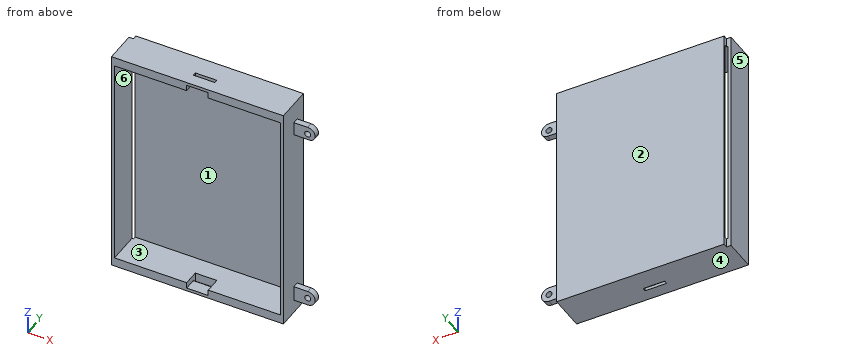
```python
from build123d import *

# Parameters (mm, degrees)
SKETCH1_R                = 1
SKETCH1_W                = 55.4
SKETCH1_H                = 71.4
BOSS_EXTRUDE1_DEPTH      = 5
SKETCH2_W                = 55.4
SKETCH2_H                = 71.4
BOSS_EXTRUDE2_DEPTH      = 1.5
SKETCH4_W                = 7.703515063
SKETCH4_H                = 8.608986158
CUT_EXTRUDE1_DEPTH       = 105.5
MOVE_FACE1_BY            = 7
MOVE_FACE2_BY            = 7.5
MOVE_FACE3_BY            = 4
MOVE_FACE3_2_BY          = 4
MOVE_FACE4_BY            = 4
MOVE_FACE4_2_BY          = 4
MOVE_FACE5_BY            = 0.4
MOVE_FACE5_2_BY          = 0.4
MOVE_FACE6_BY            = 0.4
MOVE_FACE6_2_BY          = 0.4
MOVE_START               = 3
MOVE_FACE7_OUTLINE_W     = 58.4
MOVE_FACE7_OUTLINE_H     = 74.4
MOVE_FACE7_OUTLINE_W_2   = 55.4
MOVE_FACE7_OUTLINE_H_2   = 71.4
MOVE_FACE7_DEPTH         = 2
MOVE_START_2             = -25.141552832
MOVE_FACE8_OUTLINE_W     = 0.5
MOVE_FACE8_OUTLINE_H     = 10
MOVE_FACE8_DEPTH         = 56
MOVE_START_3             = -33.2
MOVE_FACE8_2_OUTLINE_W   = 58.4
MOVE_FACE8_2_OUTLINE_H   = 10
MOVE_FACE8_2_DEPTH       = 0.5
MOVE_START_4             = 40.7
MOVE_FACE8_3_OUTLINE_W   = 58.4
MOVE_FACE8_3_OUTLINE_H   = 10
MOVE_FACE8_3_DEPTH       = 0.5
MOVE_START_5             = -32.7
MOVE_FACE8_4_OUTLINE_W   = 0.5
MOVE_FACE8_4_OUTLINE_H   = 10
MOVE_FACE8_4_OUTLINE_H_2 = 1
MOVE_FACE8_4_DEPTH       = 73.4
MOVE_START_6             = 35.858447168
MOVE_FACE8_5_OUTLINE_W   = 0.5
MOVE_FACE8_5_OUTLINE_H   = 9
MOVE_FACE8_5_DEPTH       = 4.841552832
MOVE_FACE8_6_OUTLINE_W   = 0.5
MOVE_FACE8_6_OUTLINE_H   = 9
MOVE_FACE8_6_DEPTH       = 2.558447168
CUT_EXTRUDE2_DEPTH       = 66
CUT_EXTRUDE2_DEPTH_BACK  = 64
SKETCH5_W                = 9.341764375
SKETCH5_H                = 8.237393027
CUT_EXTRUDE3_DEPTH       = 4
FILLET3_R                = 2
MOVE_FACE9_OUTLINE_W     = 57.4
MOVE_FACE9_OUTLINE_H     = 73.4
MOVE_FACE9_OUTLINE_W_2   = 55.4
MOVE_FACE9_OUTLINE_H_2   = 71.4
MOVE_FACE9_DEPTH         = 2.5
SKETCH7_W                = 57.4
SKETCH7_H                = 73.4
BOSS_EXTRUDE3_DEPTH      = 0.5
SKETCH8_W                = 57.4
SKETCH8_H                = 73.4
CUT_EXTRUDE4_DEPTH       = 1
MOVE_FACE10_BY           = 0.25
MOVE_FACE10_2_BY         = 0.25
MOVE_FACE11_BY           = 0.25
MOVE_FACE11_2_BY         = 0.25
SKETCH9_W                = 1.5
SKETCH9_H                = 73.4
CUT_EXTRUDE5_DEPTH       = 1.5
MOVE_START_7             = -34.7
MOVE_FACE12_DEPTH        = 2
MOVE_FACE12_2_DEPTH      = 2
CUT_EXTRUDE6_DEPTH       = 5.2
SKETCH12_W               = 7.2
SKETCH12_H               = 1.2
CUT_EXTRUDE7_DEPTH       = 108.2


# Read off the part's stored shape, not the designer's step: Move Face7, Move Face8, Move Face9, Move Face12
with BuildPart() as part:
    # Sketch1 → Boss-Extrude1 (new body)
    with BuildSketch(Plane(origin=(0, 0, 0), x_dir=(1, 0, 0), z_dir=(0, 1, 0))):
        with BuildLine():
            Line((26.077909727, -37.2), (26.077909727, -35.858447168))
            Line((26.077909727, -35.858447168), (29.822090273, -35.858447168))
            ThreePointArc((29.822090273, -35.858447168), (32.322090273, -33.358447168), (29.822090273, -30.858447168))
            Line((29.822090273, -30.858447168), (26.077909727, -30.858447168))
            Line((26.077909727, -30.858447168), (26.077909727, 25.141552832))
            Line((26.077909727, 25.141552832), (29.822090273, 25.141552832))
            ThreePointArc((29.822090273, 25.141552832), (32.322090273, 27.641552832), (29.822090273, 30.141552832))
            Line((29.822090273, 30.141552832), (26.077909727, 30.141552832))
            Line((26.077909727, 30.141552832), (26.077909727, 37.2))
            Line((26.077909727, 37.2), (-32.322090273, 37.2))
            Line((-32.322090273, 37.2), (-32.322090273, -37.2))
            Line((-32.322090273, -37.2), (26.077909727, -37.2))
        make_face()
        with Locations(Location((29.822090273, 27.641552832, 0), (0, 0, 270))):
            Circle(SKETCH1_R, mode=Mode.SUBTRACT)
        with Locations(Location((29.822090273, -33.358447168, 0), (0, 0, 270))):
            Circle(SKETCH1_R, mode=Mode.SUBTRACT)
        with Locations((-3.122090273, 0)):
            Rectangle(SKETCH1_W, SKETCH1_H, mode=Mode.SUBTRACT)
    extrude(amount=BOSS_EXTRUDE1_DEPTH)

    # Sketch2 → Boss-Extrude2 (add)
    with BuildSketch(Plane(origin=(0, 0, 0), x_dir=(1, 0, 0), z_dir=(0, 1, 0))):
        with Locations((-3.122090273, 0)):
            Rectangle(SKETCH2_W, SKETCH2_H)
    extrude(amount=BOSS_EXTRUDE2_DEPTH)

    # Sketch4 → Cut-Extrude1 (cut)
    with BuildSketch(Plane.XY.offset(35.858447168)):
        with Locations((29.929667259, 6.304493079)):
            Rectangle(SKETCH4_W, SKETCH4_H)
    extrude(amount=-CUT_EXTRUDE1_DEPTH, mode=Mode.SUBTRACT)

    # Move Face1: a face moved outward by 7.0
    extrude(part.faces().sort_by_distance((-2.752621979, 0, 0.033029774))[0], amount=MOVE_FACE1_BY, dir=(0, -1, 0))

    # Move Face2: a face moved inward by 7.5
    extrude(part.faces().sort_by_distance((-3.122090273, 1.5, 0))[0], amount=MOVE_FACE2_BY, dir=(0, -1, 0), mode=Mode.SUBTRACT)

    # Move Face3: a face moved outward by 4.0
    extrude(part.faces().sort_by_distance((-3.122090273, -1, 37.2))[0], amount=MOVE_FACE3_BY, dir=(0, 0, 1))

    # Move Face3 2: a face moved outward by 4.0
    extrude(part.faces().sort_by_distance((-3.122090273, -0.5, -35.7))[0], amount=MOVE_FACE3_2_BY, dir=(0, 0, 1))

    # Move Face4: a face moved inward by 4.0
    extrude(part.faces().sort_by_distance((-3.122090273, -0.5, 35.7))[0], amount=MOVE_FACE4_BY, dir=(0, 0, 1), mode=Mode.SUBTRACT)

    # Move Face4 2: a face moved inward by 4.0
    extrude(part.faces().sort_by_distance((-3.122090273, -1, -37.2))[0], amount=MOVE_FACE4_2_BY, dir=(0, 0, 1), mode=Mode.SUBTRACT)

    # Move Face5: a face moved outward by 0.4
    extrude(part.faces().sort_by_distance((24.577909727, -0.5, 4))[0], amount=MOVE_FACE5_BY, dir=(-1, 0, 0))

    # Move Face5 2: a face moved outward by 0.4
    extrude(part.faces().sort_by_distance((-32.322090273, -1, 4))[0], amount=MOVE_FACE5_2_BY, dir=(-1, 0, 0))

    # Move Face6: a face moved inward by 0.4
    extrude(part.faces().sort_by_distance((-30.822090273, -0.5, 4))[0], amount=MOVE_FACE6_BY, dir=(-1, 0, 0), mode=Mode.SUBTRACT)

    # Move Face6 2: a face moved inward by 0.4
    extrude(part.faces().sort_by_distance((26.077909727, -0.831838565, 4.127976775))[0], amount=MOVE_FACE6_2_BY, dir=(-1, 0, 0), mode=Mode.SUBTRACT)

    # Move Face7 outline → Move Face7 (cut)
    with BuildSketch(Plane(origin=(0, 0, 0), x_dir=(1, 0, 0), z_dir=(0, 1, 0)).offset(MOVE_START)):
        with Locations((-3.522090273, -4)):
            Rectangle(MOVE_FACE7_OUTLINE_W, MOVE_FACE7_OUTLINE_H)
        with Locations((-3.522090273, -4)):
            Rectangle(MOVE_FACE7_OUTLINE_W_2, MOVE_FACE7_OUTLINE_H_2, mode=Mode.SUBTRACT)
    extrude(amount=MOVE_FACE7_DEPTH, mode=Mode.SUBTRACT)

    # Move Face8 outline → Move Face8 (cut)
    with BuildSketch(Plane.XY.offset(MOVE_START_2)):
        with Locations((-32.472090273, -2)):
            Rectangle(MOVE_FACE8_OUTLINE_W, MOVE_FACE8_OUTLINE_H)
        with Locations((25.427909727, -2)):
            Rectangle(MOVE_FACE8_OUTLINE_W, MOVE_FACE8_OUTLINE_H)
    extrude(amount=MOVE_FACE8_DEPTH, mode=Mode.SUBTRACT)

    # Move Face8 2 outline → Move Face8 2 (cut)
    with BuildSketch(Plane.XY.offset(MOVE_START_3)):
        with Locations((-3.522090273, -2)):
            Rectangle(MOVE_FACE8_2_OUTLINE_W, MOVE_FACE8_2_OUTLINE_H)
    extrude(amount=MOVE_FACE8_2_DEPTH, mode=Mode.SUBTRACT)

    # Move Face8 3 outline → Move Face8 3 (cut)
    with BuildSketch(Plane.XY.offset(MOVE_START_4)):
        with Locations((-3.522090273, -2)):
            Rectangle(MOVE_FACE8_3_OUTLINE_W, MOVE_FACE8_3_OUTLINE_H)
    extrude(amount=MOVE_FACE8_3_DEPTH, mode=Mode.SUBTRACT)

    # Move Face8 4 outline → Move Face8 4 (cut)
    with BuildSketch(Plane.XY.offset(MOVE_START_5)):
        with Locations((-32.472090273, -2)):
            Rectangle(MOVE_FACE8_4_OUTLINE_W, MOVE_FACE8_4_OUTLINE_H)
        with Locations((25.427909727, 2.5)):
            Rectangle(MOVE_FACE8_4_OUTLINE_W, MOVE_FACE8_4_OUTLINE_H_2)
    extrude(amount=MOVE_FACE8_4_DEPTH, mode=Mode.SUBTRACT)

    # Move Face8 5 outline → Move Face8 5 (cut)
    with BuildSketch(Plane.XY.offset(MOVE_START_6)):
        with Locations((25.427909727, -2.5)):
            Rectangle(MOVE_FACE8_5_OUTLINE_W, MOVE_FACE8_5_OUTLINE_H)
    extrude(amount=MOVE_FACE8_5_DEPTH, mode=Mode.SUBTRACT)

    # Move Face8 6 outline → Move Face8 6 (cut)
    with BuildSketch(Plane.XY.offset(MOVE_START_5)):
        with Locations((25.427909727, -2.5)):
            Rectangle(MOVE_FACE8_6_OUTLINE_W, MOVE_FACE8_6_OUTLINE_H)
    extrude(amount=MOVE_FACE8_6_DEPTH, mode=Mode.SUBTRACT)

    # Sketch5 → Cut-Extrude2 (cut, two sides: drawn at the far end of the back side and taken through both)
    with BuildSketch(Plane.XY.offset(-CUT_EXTRUDE2_DEPTH_BACK)):
        with Locations((29.848791915, -4.118696514)):
            Rectangle(SKETCH5_W, SKETCH5_H)
    extrude(amount=CUT_EXTRUDE2_DEPTH + CUT_EXTRUDE2_DEPTH_BACK, mode=Mode.SUBTRACT)

    # Sketch6 → Cut-Extrude3 (cut)
    with BuildSketch(Plane(origin=(0, 2, 0), x_dir=(1, 0, 0), z_dir=(0, 1, 0))):
        Polygon((25.177909727, -30.858447168), (25.177909727, -31.358447168), (32.688438313, -31.358447168), (32.688438313, -30.19770306), (25.177909727, -30.19770306), align=None)
    extrude(amount=-CUT_EXTRUDE3_DEPTH, mode=Mode.SUBTRACT)

    # Fillet3
    fillet3_edges = [part.edges().sort_by_distance(p)[0] for p in [
        (31.322090273, 1, 31.358447168),
    ]]
    fillet(fillet3_edges, radius=FILLET3_R)

    # Move Face9 outline → Move Face9 (add)
    with BuildSketch(Plane(origin=(0, 0, 0), x_dir=(1, 0, 0), z_dir=(0, 1, 0)).offset(MOVE_START)):
        with Locations((-3.522090273, -4)):
            Rectangle(MOVE_FACE9_OUTLINE_W, MOVE_FACE9_OUTLINE_H)
        with Locations((-3.522090273, -4)):
            Rectangle(MOVE_FACE9_OUTLINE_W_2, MOVE_FACE9_OUTLINE_H_2, mode=Mode.SUBTRACT)
    extrude(amount=MOVE_FACE9_DEPTH)

    # Sketch7 → Boss-Extrude3 (add)
    with BuildSketch(Plane(origin=(0, 5.5, 0), x_dir=(1, 0, 0), z_dir=(0, 1, 0))):
        with Locations((-3.522090273, -4)):
            Rectangle(SKETCH7_W, SKETCH7_H)
    extrude(amount=BOSS_EXTRUDE3_DEPTH)

    # Sketch8 → Cut-Extrude4 (cut)
    with BuildSketch(Plane.XZ.offset(7)):
        with Locations((-3.522090273, 4)):
            Rectangle(SKETCH8_W, SKETCH8_H)
    extrude(amount=-CUT_EXTRUDE4_DEPTH, mode=Mode.SUBTRACT)

    # Move Face10: a face moved inward by 0.25
    extrude(part.faces().sort_by_distance((28.366938403, 0, -27.641552832))[0], amount=MOVE_FACE10_BY, dir=(0, 1, 0), mode=Mode.SUBTRACT)

    # Move Face10 2: a face moved inward by 0.25
    extrude(part.faces().sort_by_distance((28.373500925, 0, 33.610852536))[0], amount=MOVE_FACE10_2_BY, dir=(0, 1, 0), mode=Mode.SUBTRACT)

    # Move Face11: a face moved outward by 0.25
    extrude(part.faces().sort_by_distance((28.373500925, 2, 33.610852536))[0], amount=MOVE_FACE11_BY, dir=(0, 1, 0))

    # Move Face11 2: a face moved outward by 0.25
    extrude(part.faces().sort_by_distance((28.366938403, 2, -27.641552832))[0], amount=MOVE_FACE11_2_BY, dir=(0, 1, 0))

    # Sketch9 → Cut-Extrude5 (cut)
    with BuildSketch(Plane(origin=(0, 6, 0), x_dir=(1, 0, 0), z_dir=(0, 1, 0))):
        with Locations((-31.472090273, -4)):
            Rectangle(SKETCH9_W, SKETCH9_H)
    extrude(amount=-CUT_EXTRUDE5_DEPTH, mode=Mode.SUBTRACT)

    # Move Face12 outline → Move Face12 (add)
    with BuildSketch(Plane.XY.offset(MOVE_START_7)):
        Polygon((-32.222090273, 4.5), (-32.222090273, -6), (25.177909727, -6), (25.177909727, 6), (-30.722090273, 6), (-30.722090273, 4.5), align=None)
    extrude(amount=MOVE_FACE12_DEPTH)

    # Move Face12 2 outline → Move Face12 2 (add)
    with BuildSketch(Plane.XY.offset(MOVE_START_4)):
        Polygon((-32.222090273, 4.5), (-32.222090273, -6), (25.177909727, -6), (25.177909727, 6), (-30.722090273, 6), (-30.722090273, 4.5), align=None)
    extrude(amount=MOVE_FACE12_2_DEPTH)

    # Sketch10 → Cut-Extrude6 (cut)
    with BuildSketch(Plane.XZ.offset(6)):
        Polygon((-3.522090273, 41.7), (0.077909727, 41.7), (0.077909727, 38.920271818), (-7.122090273, 38.920271818), (-7.122090273, 41.7), align=None)
        Polygon((-7.122090273, -33.7), (-3.522090273, -33.7), (0.077909727, -33.7), (0.077909727, -30.920271818), (-7.122090273, -30.920271818), align=None)
    extrude(amount=-CUT_EXTRUDE6_DEPTH, mode=Mode.SUBTRACT)

    # Sketch12 → Cut-Extrude7 (cut)
    with BuildSketch(Plane.XY.offset(42.7)):
        with Locations((-3.522090273, -1.4)):
            Rectangle(SKETCH12_W, SKETCH12_H)
    extrude(amount=-CUT_EXTRUDE7_DEPTH, mode=Mode.SUBTRACT)


solid = part.part
```
Source: CAD feature listing. Evaluate the final solid. Frame: model axes, mm. Face numbers are marked on the shaded views. A direction names the side the tool comes from. Give positions to 0.01 mm unless a question says otherwise; leave off trailing zeros. Order: outer loops, then holes, each group sorted by start corner. A loop starts at its lowest first (then second) coordinate and runs counter-clockwise, first axis right, second up. Notation, with made-up numbers: (26, -31) -> (61, -31) arc R29 cw to (61, -9) -> close; hole circle Ø6 at (72.5, 36.25). An arc over 180 degrees is marked (long way). Use a Markdown table: item, result.
Q1. Section D-D (x = -6). Return the cut outline in (y, z), and give its area (3 significant figures).
A:
| item | result |
|---|---|
| outline | (-6, -34.7) -> (-2, -34.7) -> (-2, -33.7) -> (-6, -33.7) -> close; (-6, 41.7) -> (-2, 41.7) -> (-2, 42.7) -> (-6, 42.7) -> close; (-0.8, -34.7) -> (6, -34.7) -> (6, 42.7) -> (-0.8, 42.7) -> (-0.8, 39.7) -> (5.5, 39.7) -> (5.5, -31.7) -> (-0.8, -31.7) -> close |
| area | 84.5 mm^2 |
Q2. Access query for the marked faces 5 and 6. Directions: +Z, -Z, +X, -X, +Y, -Y. A direction counts if a zero-diameter tool reaches every point of the face in a straight line with its end or side. Return the directions, or none.
A:
| item | result |
|---|---|
| face 5 | +Z, -Z, -X, +Y, -Y |
| face 6 | +Y, -Y |
Q3. Section B-B (y = -3.75). Return the cut outline in (x, z), and give its area (3 significant figures).
A:
| item | result |
|---|---|
| outline | (-32.22, -34.7) -> (25.18, -34.7) -> (25.18, 42.7) -> (-32.22, 42.7) -> close; hole (-31.22, -31.7) -> (-7.12, -31.7) -> (-7.12, -33.7) -> (0.08, -33.7) -> (0.08, -31.7) -> (24.18, -31.7) -> (24.18, 39.7) -> (0.08, 39.7) -> (0.08, 41.7) -> (-7.12, 41.7) -> (-7.12, 39.7) -> (-31.22, 39.7) -> close |
| area | 458 mm^2 |
Q4. Section A-A (x = 26). Return the cut outline in (y, z).
A:
| item | result |
|---|---|
| outline | (0.25, -30.14) -> (2.25, -30.14) -> (2.25, -25.14) -> (0.25, -25.14) -> close; (0.25, 31.36) -> (2.25, 31.36) -> (2.25, 35.86) -> (0.25, 35.86) -> close |
Q5. Pull-direction query (Z, two-part tool) for the marked faces 1, 2, 3 and 4; classes: +Z half, -Z half, draft (parallel to the pull), parting line (faces both ways), or undercut.
A:
| item | result |
|---|---|
| face 1 | undercut |
| face 2 | draft |
| face 3 | undercut |
| face 4 | -Z half |
Q6. Section C-C (z = 28). Return the cut outline in (x, y), and give its area (4 significant figures).
A:
| item | result |
|---|---|
| outline | (-32.22, -6) -> (-31.22, -6) -> (-31.22, 4.5) -> (-32.22, 4.5) -> close; (-30.72, 5.5) -> (24.18, 5.5) -> (24.18, -6) -> (25.18, -6) -> (25.18, 6) -> (-30.72, 6) -> close |
| area | 49.95 mm^2 |
Q7. First-contact query: P1, Ø2, axis at x = 5.5, z = 27.5, coming from the -Y side; P2, Ø1.6, axis at x = 29.82, z = -27.64, coming from the -Y side; P3, Ø2.5, axis at y = -4, z = 41, coming from the +X side; P4, Ø1, axis at x = 27.5, y = 1.5, coming from the +Z side. Flat tips, straight axial feed; report the tip coordinate or a pass-through.
A:
| item | result |
|---|---|
| P1 | y = 5.5 |
| P2 | through |
| P3 | x = 25.18 |
| P4 | z = 35.86 |
Q8. Material intervals for line 1 (Z direction, x = 5, y = 0.25); line 2 (X direction, y = -1.5, z = 19); line 3 (Y direction, x = -12, z = -27), sorted ascending. Write a range as [from, to].
A:
| item | result |
|---|---|
| line 1 | [-34.7, -31.7], [39.7, 42.7] |
| line 2 | [-32.22, -31.22], [24.18, 25.18] |
| line 3 | [5.5, 6] |
